```python
from build123d import *

# Parameters (mm, degrees)
SKETCH1_R           = 1.5
SKETCH1_R_2         = 32.5
BOSS_EXTRUDE1_DEPTH = 2
BOSS_EXTRUDE2_DEPTH = 2


with BuildPart() as part:
    # Sketch1 → Boss-Extrude1 (new body)
    with BuildSketch(Plane(origin=(12.910322113, 55.576390481, 0), x_dir=(0.974063756, -0.226273724, 0), z_dir=(0.226273724, 0.974063756, 0))):
        with BuildLine():
            Line((-65.421780539, -70.276441512), (-3.421780539, -70.276441512))
            ThreePointArc((-3.421780539, -70.276441512), (0.113753366, -68.811975418), (1.578219461, -65.276441512))
            Line((1.578219461, -65.276441512), (1.578219461, -3.276441512))
            ThreePointArc((1.578219461, -3.276441512), (0.113753366, 0.259092394), (-3.421780539, 1.723558488))
            Line((-3.421780539, 1.723558488), (-65.421780539, 1.723558488))
            ThreePointArc((-65.421780539, 1.723558488), (-68.957314445, 0.259092394), (-70.421780539, -3.276441512))
            Line((-70.421780539, -3.276441512), (-70.421780539, -65.276441512))
            ThreePointArc((-70.421780539, -65.276441512), (-68.957314445, -68.811975418), (-65.421780539, -70.276441512))
        make_face()
        with Locations((-65.171780539, -3.526441512)):
            Circle(SKETCH1_R, mode=Mode.SUBTRACT)
        with Locations((-65.171780539, -65.026441512)):
            Circle(SKETCH1_R, mode=Mode.SUBTRACT)
        with Locations((-3.671780539, -65.026441512)):
            Circle(SKETCH1_R, mode=Mode.SUBTRACT)
        with Locations((-3.671780539, -3.526441512)):
            Circle(SKETCH1_R, mode=Mode.SUBTRACT)
        with Locations((-34.421780539, -34.276441512)):
            Circle(SKETCH1_R_2, mode=Mode.SUBTRACT)
    extrude(amount=BOSS_EXTRUDE1_DEPTH)

    # Sketch2 → Boss-Extrude2 (add)
    with BuildSketch(Plane(origin=(13.362869562, 57.524517994, 0), x_dir=(0.974063756, -0.226273724, 0), z_dir=(0.226273724, 0.974063756, 0))):
        with BuildLine():
            Line((-2.060538289, -31.276441512), (-31.421780539, -31.276441512))
            Line((-31.421780539, -31.276441512), (-31.421780539, -1.915199262))
            ThreePointArc((-31.421780539, -1.915199262), (-57.402750928, -57.257411901), (-2.060538289, -31.276441512))
        make_face()
    extrude(amount=-BOSS_EXTRUDE2_DEPTH)


solid = part.part
```
Here's how the part is built. I have some questions about the finished solid (model axes, mm). Coordinates: 2 decimals unless noted, no trailing zeros. Write each loop counter-clockwise with the first axis right and the second up, starting at its lowest first coordinate (ties: lowest second). Pieces come first, ordered by that corner, then holes. Notation, with made-up numbers: (14, 47) -> (51, 47) arc R17 ccw to (51, 63) -> close; hole circle Ø11 at (-7.75, 62). An arc over 180 degrees is marked (long way). Use a Markdown table: item, result. Add a question column.
(1) If we section it at C-C, the plane x = -28: Write out the boundary of the cut face in (y, z).
(2) We'd pull the mould along Z, two halves only. Please class faces 1 (the cylindrical face through (-54.073, 72.149, 68.773)), 2 (the flat face through (-20, 64, -1.724)), 3 (the flat face through (-20.66, 65.43, 33.77)), 4 (the flat face through (-17.47, 63.67, 16.8)): +Z half, -Z half, draft (parallel to the pull), parting line (faces both ways), or undercut.
(3) If we section it at A-A, the plane z = 15: Write out the boundary of the cut face in (x, y).
(4) I'm going to push flat-ended pins straight in: P1, Ø3, axis at x = -36, y = 64.5, coming from the +Z side; P2, Ø8, axis at x = -27, y = 64, coming from the +Z side. Where does each tip first touch, or does it pass through?
(5) If we section it at B-B, the plane z = 59.5: Write out the boundary of the cut face in (x, y).
(6) Please list where these lines run through material, in increasing order: line 1 (X direction, y = 57, z = 29.5); line 2 (Y direction, x = -15.5, z = 54); line 3 (Y direction, x = -1.5, z = 39.5).
Outcome:
| question | item | result |
|---|---|---|
| 1 | outline | (65.08, -1.72) -> (67.13, -1.72) -> (67.13, 70.28) -> (65.08, 70.28) -> close |
| 2 | face 1 | +Z half |
| 2 | face 2 | -Z half |
| 2 | face 3 | draft |
| 2 | face 4 | undercut |
| 3 | outline | (-55.68, 71.51) -> (-17.7, 62.69) -> (-17.24, 64.63) -> (-55.23, 73.46) -> close; (4.87, 57.44) -> (14.45, 55.22) -> (14.9, 57.17) -> (5.32, 59.39) -> close |
| 4 | P1 | passes through |
| 4 | P2 | stops at z = 70.28 |
| 5 | outline | (-55.68, 71.51) -> (14.45, 55.22) -> (14.9, 57.17) -> (-55.23, 73.46) -> close |
| 6 | line 1 | x = 10.91 to 14.86 |
| 6 | line 2 | y = 62.18 to 64.23 |
| 6 | line 3 | y = 58.92 to 60.98 |
